Part model, mm, in its own coordinate system. Face numbers are marked on the shaded views. A direction names the side the tool comes from. Round coordinates to 2 decimals unless told otherwise and drop trailing zeros. Write each loop counter-clockwise with the first axis right and the second up, starting at its lowest first coordinate (ties: lowest second). Pieces come first, ordered by that corner, then holes.
Autodesk Inventor part; units mm, degrees
ref_plane "Start Plane" through (0, 0, 0) normal (1, 0, 0) x (0, 1, 0)
ref_plane "XZ Plane" through (0, 0, 0) normal (0, 1, 0) x (-1, 0, 0)
ref_plane "XY Plane" through (0, 0, 0) normal (0, 0, 1) x (1, 0, 0)
sketch "Main Sketch" plane through (0, 0, 0) normal (0, 0, 1) x (1, 0, 0)
  line L0 (0, 0) -> (15, 0)
  line L1 (0, 0) -> (0, 3.5)
  line L2 (0, 3.5) -> (4, 3.5)
  line L3 (4, 3.5) -> (4, 6)
  line L4 (11, 6) -> (11, 3.5)
  line L5 (4, 6) -> (11, 6)
  line L6 (15, 3.5) -> (15, 0)
  line L7 (11, 3.5) -> (15, 3.5)
  dimension "d3" = 7
  dimension "d4" = 12
  dimension "d5" = 7
revolve "Revolution1" add sketch "Main Sketch" angle 360 about axis through (0, 0, 0) along (1, 0, 0)
sketch "Sketch3" plane through (0, 0, 0) normal (-1, 0, 0) x (0, 0, 1)
  circle A0 centre (0, 0) radius 1.5
  dimension "d7" = 3
extrude "Extrusion1" cut sketch "Sketch3" against normal up to surface (15 mm away)
equation "\"Length\" = 15"
properties part number "Shaft" material "Steel"
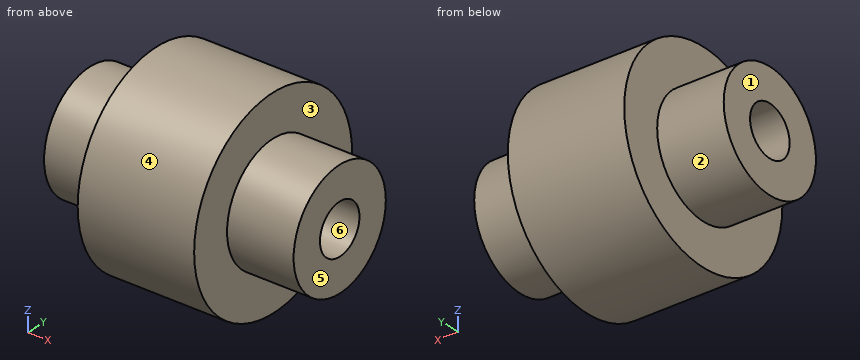
Q1. Drop flat-ended pins along their axis: P1, Ø1, axis at x = 13.5, y = -3.5, coming from the -Z side; P2, Ø2, axis at x = 3.5, y = 4, coming from the -Z side; P3, Ø1.5, axis at x = 3.5, y = 2, coming from the +Z side. Give the stop position or say it passes through.
Q2. Wall check: line 1 (X direction, y = 2.75, z = -4.25); line 2 (Z direction, x = 13, y = -3); line 3 (Z direction, x = 1.5, y = -1.25). Give the ranges that are in metal, low to high.
Q3. Two-plate mould, pull along Y, no slides. Class the marked faces 4, 5 and 6: released by +Y, released by -Y, zero draft, split by the parting line, or undercut.
Q4. Tool access for the marked faces 1, 2 and 3: list every direction of +Z, -Z, +X, -X, +Y, -Y with a clear straight run to the whole face (end or side of a thin tool).
Q5. Saw through at A-A, the plane y = 0. Write the cut outline in (x, z), and give its area (3 significant figures).
Q6. Saw through at C-C, the plane x = 2. Write the cut outline in (y, z), and give its area (3 significant figures).
Q7. Saw through at D-D, the plane z = -2.75. Write the cut outline in (x, y), and give its area (3 significant figures).
Computed:
1. P1: stops at z = -1.8
1. P2: stops at z = -5.12
1. P3: stops at z = 5.82
2. line 1: x = 4 to 11
2. line 2: z = -1.8 to 1.8
2. line 3: z = -3.27 to -0.83, 0.83 to 3.27
3. face 4: split by the parting line
3. face 5: zero draft
3. face 6: undercut
4. face 1: +Z, -Z, -X, +Y, -Y
4. face 2: -X
4. face 3: +X
5. outline: (0, -3.5) - (4, -3.5) - (4, -6) - (11, -6) - (11, -3.5) - (15, -3.5) - (15, -1.5) - (0, -1.5) - close; (0, 1.5) - (15, 1.5) - (15, 3.5) - (11, 3.5) - (11, 6) - (4, 6) - (4, 3.5) - (0, 3.5) - close
5. area: 95.0 mm2
6. outline: circle Ø7 at (0, 0); hole circle Ø3 at (0, 0)
6. area: 31.4 mm2
7. outline: (0, -2.17) - (4, -2.17) - (4, -5.33) - (11, -5.33) - (11, -2.17) - (15, -2.17) - (15, 2.17) - (11, 2.17) - (11, 5.33) - (4, 5.33) - (4, 2.17) - (0, 2.17) - close
7. area: 109 mm2
